Here's the drawing with two shaded views (mm, measured from the low corner). I have some questions. Coordinates: 2 decimals unless noted, no trailing zeros. Order: outer loops, then holes, each group sorted by start corner. A loop starts at its lowest first (then second) coordinate and runs counter-clockwise, first axis right, second up. Notation, with made-up numbers: (20, 69) -> (24, 69) arc R21 cw to (24, 76) -> close; hole circle Ø8 at (-19.5, 12). An arc over 180 degrees is marked (long way). Write item = value, one per line.
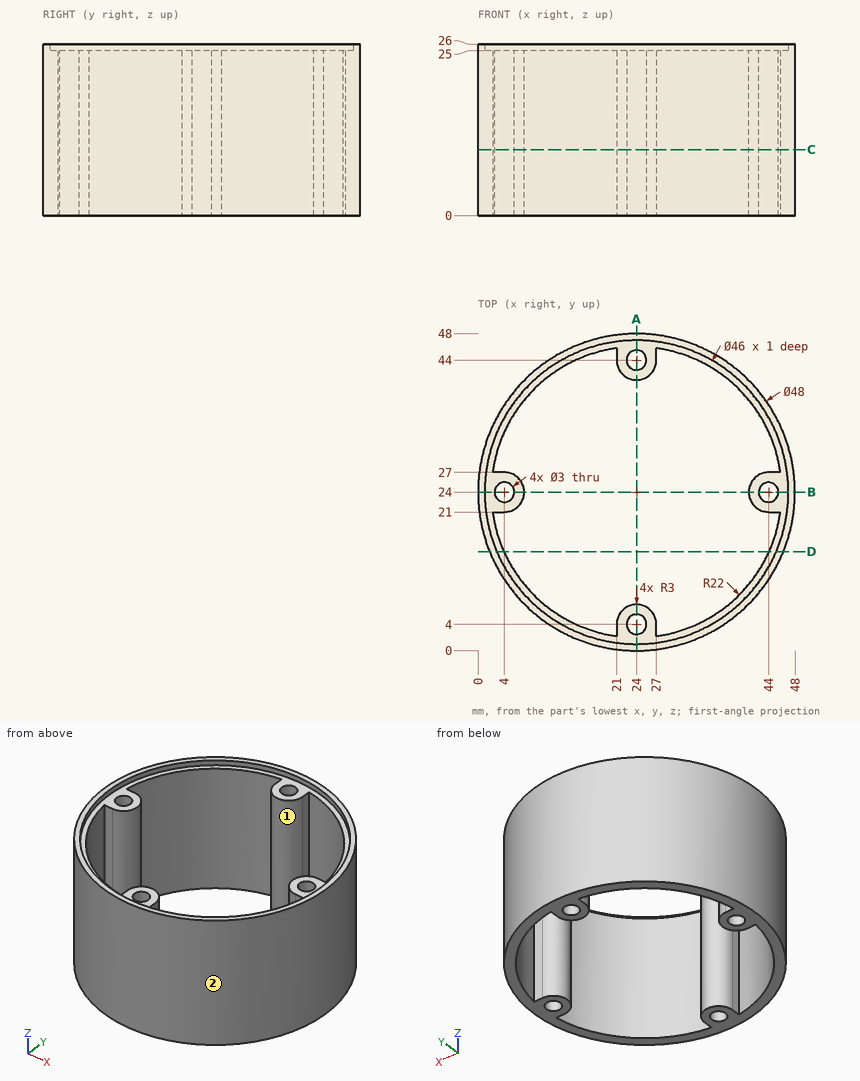
Item 1: I want a section at D-D, the plane y = 15. Please give me the cut outline in (x, z).
A:
outline = (1.75, 0) -> (3.93, 0) -> (3.93, 25) -> (2.83, 25) -> (2.83, 26) -> (1.75, 26) -> close; (44.07, 0) -> (46.25, 0) -> (46.25, 26) -> (45.17, 26) -> (45.17, 25) -> (44.07, 25) -> close
Item 2: I'm going to push flat-ended pins straight in: P1, Ø2, axis at y = 45, z = 13, coming from the +X side; P2, Ø5, axis at x = 44, y = 24, coming from the +Z side; P3, Ø12, axis at x = 35, z = 9.5, coming from the -Y side. Where does each tip first touch, or does it pass through?
A:
P1 = 37.27
P2 = 25
P3 = 0.53
Item 3: If we mould it in two halves opening along Y, with no side actions, what happens to the marked faces 1 and 2? For each: pulls with the +Y half, pulls with the -Y half, needs draft (parallel to the pull), parting line crosses it, or undercut.
A:
face_1 = undercut
face_2 = parting line crosses it
Item 4: I want a section at A-A, the plane x = 24. Please give me the cut outline in (y, z).
A:
outline = (0, 0) -> (2.5, 0) -> (2.5, 25) -> (1, 25) -> (1, 26) -> (0, 26) -> close; (5.5, 0) -> (7, 0) -> (7, 25) -> (5.5, 25) -> close; (41, 0) -> (42.5, 0) -> (42.5, 25) -> (41, 25) -> close; (45.5, 0) -> (48, 0) -> (48, 26) -> (47, 26) -> (47, 25) -> (45.5, 25) -> close
Item 5: I want a section at C-C, the plane z = 10. Please give me the cut outline in (x, y), plus the area to 3 significant figures.
A:
outline = circle Ø48 at (24, 24); hole (2.21, 21) arc R22 ccw to (21, 2.21) -> (21, 4) arc R3 cw to (27, 4) -> (27, 2.21) arc R22 ccw to (45.79, 21) -> (44, 21) arc R3 cw to (44, 27) -> (45.79, 27) arc R22 ccw to (27, 45.79) -> (27, 44) arc R3 cw to (21, 44) -> (21, 45.79) arc R22 ccw to (2.21, 27) -> (4, 27) arc R3 cw to (4, 21) -> close; hole circle Ø3 at (4, 24); hole circle Ø3 at (24, 4); hole circle Ø3 at (24, 44); hole circle Ø3 at (44, 24)
area = 364 mm2
Item 6: If I drill on probe 1 along Y at (x, z) = (24, 4.5); probe 2 along X at (y, z) = (5, 19.5); probe 3 along Z at (x, y) = (45, 32), over which ranges is the centre line in solid material (lowest first)?
A:
probe_1 = 0 to 2.5, 5.5 to 7, 41 to 42.5, 45.5 to 48
probe_2 = 9.34 to 12.91, 21.17 to 22.88, 25.12 to 26.83, 35.09 to 38.66
probe_3 = 0 to 25
